The model under review builds one solid part; all positions refer to its coordinate system, in mm. Face numbers are marked on the shaded views. A direction names the side the tool comes from. Round coordinates to 2 decimals unless told otherwise and drop trailing zeros. Loops run counter-clockwise (first coordinate to the right, second up) from the corner with the lowest first, then second, coordinate; pieces in that order, holes last. Notation, with made-up numbers: M 12.5,-27.5 L 59.5,-27.5 A19 ccw 59.5,-10.5 Z; hole C 13.5,15.5 d11. An arc over 180 degrees is marked long. Return JSON: item names as keys, results as strings. Group by question number.
Q1. Consider section B-B (z = 104). State the section outline as (x, y) points.
Q2. Consider section A-A (y = -46). State the section outline as (x, z) points, and give its area (3 significant figures).
Q3. Clearance check with flat-ended pins moving along their axes: pin 1 Ø10 at (x, z) = (64, 20) entering from +Y; pin 2 Ø1 at (y, z) = (-5.5, 38.5) entering from -X; pin 3 Ø7 at (y, z) = (-6, 104) entering from -X; pin 4 Ø1 at (y, z) = (-14, 52.5) entering from +X. State where each tip first meets the part, or that it passes through.
Q4. Draft analysis for pull direction Y (two halves, no side actions). For the marked faces 1, 2, 3 and 4, state which applies: pulls with the +Y half, pulls with the -Y half, needs draft (parallel to the pull), parting line crosses it, or undercut.
Q5. For the marked faces 5, 6 and 7, list the 3-axis set-ups (+Z, -Z, +X, -X, +Y, -Y) from which the entire face can be reached by the end or side of a thin tool; tool diameter is ignored.
Q6. Consider section D-D (z = 83). State the section outline as (x, y) points, and give its area (3 significant figures).
Q7. Consider section C-C (x = 46). State the section outline as (y, z) points.
Q8. To check wall thickness, follow line 1 along Z through (x, y) = (66.25, -46); line 2 along Y through (x, z) = (32, 87); line 3 along X through (y, z) = (-8.5, 64.5). State the ranges of each line that lie inside material, in increasing order.
from build123d import *

# Parameters (mm, degrees)
F1_DEPTH      = 52
F2_W          = 63
F2_H          = 28
F3_DEPTH      = 110.001
F3_DEPTH_BACK = 20.001
F4_R          = 2.75
F5_DEPTH      = 12.001


with BuildPart() as f1:
    # F0 (on Front) → F1 (new body)
    with BuildSketch(Plane.XZ):
        Polygon((0, 12), (0, 0), (63, 0), (63, -20), (75, -20), (75, 0), (75, 12), (12, 12), (12, 78), (75, 78), (75, 90), (75, 110), (63, 110), (63, 90), (0, 90), align=None)
    extrude(amount=F1_DEPTH)

    # F2 (on face) → F3 (cut, two sides)
    with BuildSketch(Plane.XY.offset(90)) as f3_sk:
        with Locations((43.5, -26)):
            Rectangle(F2_W, F2_H)
    extrude(amount=-F3_DEPTH, mode=Mode.SUBTRACT)
    extrude(f3_sk.sketch, amount=F3_DEPTH_BACK, mode=Mode.SUBTRACT)

    # F4 (on face) → F5 (cut, through all)
    with BuildSketch(Plane(origin=(63, 0, 0), x_dir=(0, -1, 0), z_dir=(-1, 0, 0))):
        with Locations((6, 104)):
            Circle(F4_R)
        with Locations((46, 104)):
            Circle(F4_R)
        with Locations((6, -14)):
            Circle(F4_R)
        with Locations((46, -14)):
            Circle(F4_R)
    extrude(amount=-F5_DEPTH, mode=Mode.SUBTRACT)


solid = f1.part
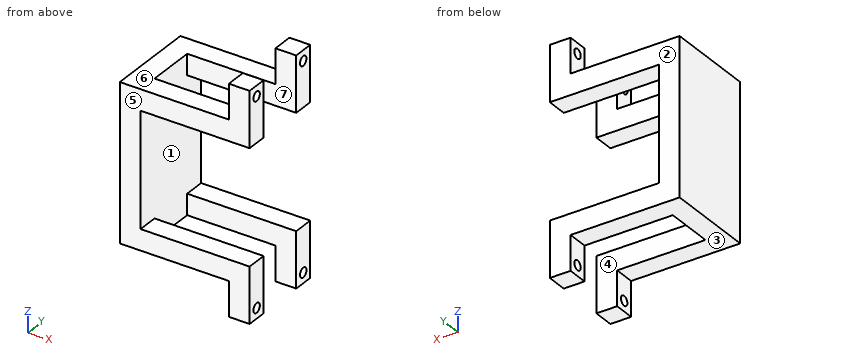
Values:
{
 "1": {"outline": "M 63,-52 L 75,-52 L 75,-48.75 L 63,-48.75 Z; M 63,-43.25 L 75,-43.25 L 75,-40 L 63,-40 Z; M 63,-12 L 75,-12 L 75,-8.75 L 63,-8.75 Z; M 63,-3.25 L 75,-3.25 L 75,0 L 63,0 Z"},
 "2": {"outline": "M 0,0 L 63,0 L 63,-11.25 L 75,-11.25 L 75,12 L 12,12 L 12,78 L 75,78 L 75,101.25 L 63,101.25 L 63,90 L 0,90 Z; M 63,-20 L 75,-20 L 75,-16.75 L 63,-16.75 Z; M 63,106.75 L 75,106.75 L 75,110 L 63,110 Z", "area": "2,940 mm2"},
 "3": {"pin 1": "passes through", "pin 2": "stops at x = 0", "pin 3": "stops at x = 63", "pin 4": "stops at x = 12"},
 "4": {"face 1": "undercut", "face 2": "pulls with the +Y half", "face 3": "needs draft", "face 4": "undercut"},
 "5": {"face 5": "+Z, -Z, +X, -X, -Y", "face 6": "+Z, -X, +Y, -Y", "face 7": "+Z, -Z, +X"},
 "6": {"outline": "M 0,-52 L 75,-52 L 75,-40 L 12,-40 L 12,-12 L 75,-12 L 75,0 L 0,0 Z", "area": "2,140 mm2"},
 "7": {"outline": "M -52,0 L -40,0 L -40,12 L -52,12 Z; M -52,78 L -40,78 L -40,90 L -52,90 Z; M -12,0 L 0,0 L 0,12 L -12,12 Z; M -12,78 L 0,78 L 0,90 L -12,90 Z"},
 "8": {"line 1": "z = -20 to -16.75, -11.25 to 12, 78 to 101.25, 106.75 to 110", "line 2": "y = -52 to -40, -12 to 0", "line 3": "x = 0 to 12"}
}
